Work out the finished part from the listing and answer in its coordinate system (mm). A direction names the side the tool comes from. Coordinates: 2 decimals unless noted, no trailing zeros. Write each loop counter-clockwise with the first axis right and the second up, starting at its lowest first coordinate (ties: lowest second). Pieces come first, ordered by that corner, then holes. Notation, with made-up numbers: (57, 24.25) - (62, 24.25) arc R35 ccw to (62, 57.25) - close; hole circle Ø10 at (-21.75, 39). An arc over 180 degrees is marked (long way). One line per item, written item: value.
```python
from build123d import *

# Parameters (mm, degrees)
ESQUISSE1_W              = 57
ESQUISSE1_H              = 57
BOSS_EXTRU_1_DEPTH       = 18.5
ESQUISSE2_W              = 51
ESQUISSE2_H              = 51
ENL_V_MAT_EXTRU_1_DEPTH  = 15.5
ESQUISSE4_W              = 10
ESQUISSE4_H              = 8
BOSS_EXTRU_2_DEPTH       = 10
ESQUISSE5_W              = 10
ESQUISSE5_H              = 8
BOSS_EXTRU_3_DEPTH       = 10
ESQUISSE6_W              = 10
ESQUISSE6_H              = 7
BOSS_EXTRU_4_DEPTH       = 10
ESQUISSE7_W              = 10
ESQUISSE7_H              = 7
BOSS_EXTRU_5_DEPTH       = 10
ESQUISSE8_R              = 1.7
ENL_V_MAT_EXTRU_2_DEPTH  = 12
ESQUISSE9_R              = 1.7
ENL_V_MAT_EXTRU_3_DEPTH  = 12
ESQUISSE16_R             = 1.7
ENL_V_MAT_EXTRU_9_DEPTH  = 12
ESQUISSE17_R             = 1.7
ENL_V_MAT_EXTRU_10_DEPTH = 12
ESQUISSE21_W             = 7.8
ESQUISSE21_H             = 2.8
ENL_V_MAT_EXTRU_14_DEPTH = 3
ENL_V_START              = -7.5
ENL_V_MAT_EXTRU_18_DEPTH = 2.7
ENL_V_MAT_EXTRU_20_DEPTH = 2.7
ESQUISSE26_W             = 5.54
ESQUISSE26_H             = 2.5
ENL_V_MAT_EXTRU_21_DEPTH = 2.847955181
ENL_V_MAT_EXTRU_22_DEPTH = 2.7
ENL_V_MAT_EXTRU_24_DEPTH = 2.7
ESQUISSE23_W             = 5.54
ESQUISSE23_H             = 2.5
ENL_V_MAT_EXTRU_26_DEPTH = 2
ESQUISSE31_W             = 5.54
ESQUISSE31_H             = 2.5
ENL_V_MAT_EXTRU_27_DEPTH = 2
ESQUISSE30_W             = 5.54
ESQUISSE30_H             = 2.5
ENL_V_MAT_EXTRU_28_DEPTH = 2
ESQUISSE32_W             = 57
ESQUISSE32_H             = 1
ENL_V_MAT_EXTRU_29_DEPTH = 0.5
ESQUISSE33_W             = 57
ESQUISSE33_H             = 1
ENL_V_MAT_EXTRU_30_DEPTH = 0.5
ESQUISSE34_W             = 57
ESQUISSE34_H             = 1
ENL_V_MAT_EXTRU_31_DEPTH = 0.5
ESQUISSE35_W             = 57
ESQUISSE35_H             = 1
ENL_V_MAT_EXTRU_32_DEPTH = 0.5
ESQUISSE36_W             = 11.4
ESQUISSE36_H             = 10.780005484
ENL_V_MAT_EXTRU_33_DEPTH = 2
CONG_1_R                 = 0.5
CONG_2_R                 = 0.5
CONG_3_R                 = 0.5
CONG_4_R                 = 0.5
CONG_5_R                 = 0.5
CONG_6_R                 = 0.5
CONG_7_R                 = 0.5
CONG_8_R                 = 0.5
CONG_9_R                 = 0.5
CONG_10_R                = 0.5
CONG_11_R                = 0.5
CONG_12_R                = 0.5
ESQUISSE38_W             = 28
ESQUISSE38_H             = 4.913001224
ENL_V_MAT_EXTRU_34_DEPTH = 3


with BuildPart() as part:
    # Esquisse1 → Boss.-Extru.1 (new body)
    with BuildSketch(Plane(origin=(0, 0, 0), x_dir=(1, 0, 0), z_dir=(0, 1, 0))):
        with Locations((-1.510072399, 8.394175698)):
            Rectangle(ESQUISSE1_W, ESQUISSE1_H)
    extrude(amount=BOSS_EXTRU_1_DEPTH)

    # Esquisse2 → Enlèv. mat.-Extru.1 (cut)
    with BuildSketch(Plane(origin=(0, 18.5, 0), x_dir=(1, 0, 0), z_dir=(0, 1, 0))):
        with Locations((-1.510072399, 8.394175698)):
            Rectangle(ESQUISSE2_W, ESQUISSE2_H)
    extrude(amount=-ENL_V_MAT_EXTRU_1_DEPTH, mode=Mode.SUBTRACT)

    # Esquisse4 → Boss.-Extru.2 (add)
    with BuildSketch(Plane(origin=(0, 3, 0), x_dir=(1, 0, 0), z_dir=(0, 1, 0))):
        with Locations((-22.010072399, 29.894175698)):
            Rectangle(ESQUISSE4_W, ESQUISSE4_H)
    extrude(amount=BOSS_EXTRU_2_DEPTH)

    # Esquisse5 → Boss.-Extru.3 (add)
    with BuildSketch(Plane(origin=(0, 3, 0), x_dir=(1, 0, 0), z_dir=(0, 1, 0))):
        with Locations((18.989927601, 29.894175698)):
            Rectangle(ESQUISSE5_W, ESQUISSE5_H)
    extrude(amount=BOSS_EXTRU_3_DEPTH)

    # Esquisse6 → Boss.-Extru.4 (add)
    with BuildSketch(Plane(origin=(0, 3, 0), x_dir=(1, 0, 0), z_dir=(0, 1, 0))):
        with Locations((18.989927601, -13.605824302)):
            Rectangle(ESQUISSE6_W, ESQUISSE6_H)
    extrude(amount=BOSS_EXTRU_4_DEPTH)

    # Esquisse7 → Boss.-Extru.5 (add)
    with BuildSketch(Plane(origin=(0, 3, 0), x_dir=(1, 0, 0), z_dir=(0, 1, 0))):
        with Locations((-22.010072399, -13.605824302)):
            Rectangle(ESQUISSE7_W, ESQUISSE7_H)
    extrude(amount=BOSS_EXTRU_5_DEPTH)

    # Esquisse8 → Enlèv. mat.-Extru.2 (cut)
    with BuildSketch(Plane(origin=(0, 13, 0), x_dir=(1, 0, 0), z_dir=(0, 1, 0))):
        with Locations(Location((19.489927601, -13.105824302, 0), (0, 0, 270))):
            Circle(ESQUISSE8_R)
    extrude(amount=-ENL_V_MAT_EXTRU_2_DEPTH, mode=Mode.SUBTRACT)

    # Esquisse9 → Enlèv. mat.-Extru.3 (cut)
    with BuildSketch(Plane(origin=(0, 13, 0), x_dir=(1, 0, 0), z_dir=(0, 1, 0))):
        with Locations(Location((-22.510072399, -13.105824302, 0), (0, 0, 270))):
            Circle(ESQUISSE9_R)
    extrude(amount=-ENL_V_MAT_EXTRU_3_DEPTH, mode=Mode.SUBTRACT)

    # Esquisse16 → Enlèv. mat.-Extru.9 (cut)
    with BuildSketch(Plane(origin=(0, 13, 0), x_dir=(1, 0, 0), z_dir=(0, 1, 0))):
        with Locations(Location((-22.510072399, 28.894175698, 0), (0, 0, 270))):
            Circle(ESQUISSE16_R)
    extrude(amount=-ENL_V_MAT_EXTRU_9_DEPTH, mode=Mode.SUBTRACT)

    # Esquisse17 → Enlèv. mat.-Extru.10 (cut)
    with BuildSketch(Plane(origin=(0, 13, 0), x_dir=(1, 0, 0), z_dir=(0, 1, 0))):
        with Locations(Location((19.489927601, 28.894175698, 0), (0, 0, 270))):
            Circle(ESQUISSE17_R)
    extrude(amount=-ENL_V_MAT_EXTRU_10_DEPTH, mode=Mode.SUBTRACT)

    # Esquisse21 → Enlèv. mat.-Extru.14 (cut)
    with BuildSketch(Plane.XY.offset(20.105824302)):
        with Locations((-1.510072399, 16.07)):
            Rectangle(ESQUISSE21_W, ESQUISSE21_H)
    extrude(amount=-ENL_V_MAT_EXTRU_14_DEPTH, mode=Mode.SUBTRACT)

    # Esquisse24 → Enlèv. mat.-Extru.18 (cut)
    with BuildSketch(Plane(origin=(0, 13, 0), x_dir=(1, 0, 0), z_dir=(0, 1, 0)).offset(ENL_V_START)):
        Polygon((19.489927601, 25.694175698), (22.261208893, 27.294175698), (22.261208893, 30.494175698), (19.489927601, 32.094175698), (16.718646309, 30.494175698), (16.718646309, 27.294175698), align=None)
    extrude(amount=-ENL_V_MAT_EXTRU_18_DEPTH, mode=Mode.SUBTRACT)

    # Esquisse25 → Enlèv. mat.-Extru.20 (cut)
    with BuildSketch(Plane(origin=(0, 13, 0), x_dir=(1, 0, 0), z_dir=(0, 1, 0)).offset(ENL_V_START)):
        Polygon((16.718646309, -11.505824302), (16.718646309, -14.705824302), (19.489927601, -16.305824302), (22.261208893, -14.705824302), (22.261208893, -11.505824302), (19.489927601, -9.905824302), align=None)
    extrude(amount=-ENL_V_MAT_EXTRU_20_DEPTH, mode=Mode.SUBTRACT)

    # Esquisse26 → Enlèv. mat.-Extru.21 (cut)
    with BuildSketch(Plane(origin=(0, 0, 10.105824302), x_dir=(-1, 0, 0), z_dir=(0, 0, -1))):
        with Locations((-19.489927601, 4.25)):
            Rectangle(ESQUISSE26_W, ESQUISSE26_H)
    extrude(amount=-ENL_V_MAT_EXTRU_21_DEPTH, mode=Mode.SUBTRACT)

    # Esquisse27 → Enlèv. mat.-Extru.22 (cut)
    with BuildSketch(Plane(origin=(0, 13, 0), x_dir=(1, 0, 0), z_dir=(0, 1, 0)).offset(ENL_V_START)):
        Polygon((-19.738791107, 27.294175698), (-19.738791107, 30.494175698), (-22.510072399, 32.094175698), (-25.281353691, 30.494175698), (-25.281353691, 27.294175698), (-22.510072399, 25.694175698), align=None)
    extrude(amount=-ENL_V_MAT_EXTRU_22_DEPTH, mode=Mode.SUBTRACT)

    # Esquisse29 → Enlèv. mat.-Extru.24 (cut)
    with BuildSketch(Plane(origin=(0, 13, 0), x_dir=(1, 0, 0), z_dir=(0, 1, 0)).offset(ENL_V_START)):
        Polygon((-19.738791107, -11.505824302), (-22.510072399, -9.905824302), (-25.281353691, -11.505824302), (-25.281353691, -14.705824302), (-22.510072399, -16.305824302), (-19.738791107, -14.705824302), align=None)
    extrude(amount=-ENL_V_MAT_EXTRU_24_DEPTH, mode=Mode.SUBTRACT)

    # Esquisse23 → Enlèv. mat.-Extru.26 (cut)
    with BuildSketch(Plane.XY.offset(-25.894175698)):
        with Locations((19.489927601, 4.25)):
            Rectangle(ESQUISSE23_W, ESQUISSE23_H)
    extrude(amount=-ENL_V_MAT_EXTRU_26_DEPTH, mode=Mode.SUBTRACT)

    # Esquisse31 → Enlèv. mat.-Extru.27 (cut)
    with BuildSketch(Plane.XY.offset(-25.894175698)):
        with Locations((-22.510072399, 4.25)):
            Rectangle(ESQUISSE31_W, ESQUISSE31_H)
    extrude(amount=-ENL_V_MAT_EXTRU_27_DEPTH, mode=Mode.SUBTRACT)

    # Esquisse30 → Enlèv. mat.-Extru.28 (cut)
    with BuildSketch(Plane(origin=(0, 0, 10.105824302), x_dir=(-1, 0, 0), z_dir=(0, 0, -1))):
        with Locations((22.510072399, 4.25)):
            Rectangle(ESQUISSE30_W, ESQUISSE30_H)
    extrude(amount=-ENL_V_MAT_EXTRU_28_DEPTH, mode=Mode.SUBTRACT)

    # Esquisse32 → Enlèv. mat.-Extru.29 (cut)
    with BuildSketch(Plane.ZY.offset(30.010072399)):
        with Locations((-8.394175698, 8.219994516)):
            Rectangle(ESQUISSE32_W, ESQUISSE32_H)
    extrude(amount=-ENL_V_MAT_EXTRU_29_DEPTH, mode=Mode.SUBTRACT)

    # Esquisse33 → Enlèv. mat.-Extru.30 (cut)
    with BuildSketch(Plane.XY.offset(20.105824302)):
        with Locations((-1.510072399, 8.219994516)):
            Rectangle(ESQUISSE33_W, ESQUISSE33_H)
    extrude(amount=-ENL_V_MAT_EXTRU_30_DEPTH, mode=Mode.SUBTRACT)

    # Esquisse34 → Enlèv. mat.-Extru.31 (cut)
    with BuildSketch(Plane(origin=(26.989927601, 0, 0), x_dir=(0, 0, -1), z_dir=(1, 0, 0))):
        with Locations((8.394175698, 8.219994516)):
            Rectangle(ESQUISSE34_W, ESQUISSE34_H)
    extrude(amount=-ENL_V_MAT_EXTRU_31_DEPTH, mode=Mode.SUBTRACT)

    # Esquisse35 → Enlèv. mat.-Extru.32 (cut)
    with BuildSketch(Plane(origin=(0, 0, -36.894175698), x_dir=(-1, 0, 0), z_dir=(0, 0, -1))):
        with Locations((1.510072399, 8.219994516)):
            Rectangle(ESQUISSE35_W, ESQUISSE35_H)
    extrude(amount=-ENL_V_MAT_EXTRU_32_DEPTH, mode=Mode.SUBTRACT)

    # Esquisse36 → Enlèv. mat.-Extru.33 (cut)
    with BuildSketch(Plane.XY.offset(20.105824302)):
        with Locations((-1.510072399, 13.109997258)):
            Rectangle(ESQUISSE36_W, ESQUISSE36_H)
    extrude(amount=-ENL_V_MAT_EXTRU_33_DEPTH, mode=Mode.SUBTRACT)

    # Congé1
    cong_1_edges = [part.edges().sort_by_distance(p)[0] for p in [
        (-7.210072399, 13.609997258, 20.105824302),
    ]]
    fillet(cong_1_edges, radius=CONG_1_R)

    # Congé2
    cong_2_edges = [part.edges().sort_by_distance(p)[0] for p in [
        (4.189927601, 13.609997258, 20.105824302),
    ]]
    fillet(cong_2_edges, radius=CONG_2_R)

    # Congé3
    cong_3_edges = [part.edges().sort_by_distance(p)[0] for p in [
        (-7.210072399, 8.219994516, 19.605824302),
    ]]
    fillet(cong_3_edges, radius=CONG_3_R)

    # Congé4
    cong_4_edges = [part.edges().sort_by_distance(p)[0] for p in [
        (4.189927601, 8.219994516, 19.605824302),
    ]]
    fillet(cong_4_edges, radius=CONG_4_R)

    # Congé5
    cong_5_edges = [part.edges().sort_by_distance(p)[0] for p in [
        (26.989927601, 13.609997258, 20.105824302),
    ]]
    fillet(cong_5_edges, radius=CONG_5_R)

    # Congé6
    cong_6_edges = [part.edges().sort_by_distance(p)[0] for p in [
        (26.989927601, 3.859997258, 20.105824302),
    ]]
    fillet(cong_6_edges, radius=CONG_6_R)

    # Congé7
    cong_7_edges = [part.edges().sort_by_distance(p)[0] for p in [
        (26.989927601, 13.609997258, -36.894175698),
    ]]
    fillet(cong_7_edges, radius=CONG_7_R)

    # Congé8
    cong_8_edges = [part.edges().sort_by_distance(p)[0] for p in [
        (26.989927601, 3.859997258, -36.894175698),
    ]]
    fillet(cong_8_edges, radius=CONG_8_R)

    # Congé9
    cong_9_edges = [part.edges().sort_by_distance(p)[0] for p in [
        (-30.010072399, 13.609997258, -36.894175698),
    ]]
    fillet(cong_9_edges, radius=CONG_9_R)

    # Congé10
    cong_10_edges = [part.edges().sort_by_distance(p)[0] for p in [
        (-30.010072399, 3.859997258, -36.894175698),
    ]]
    fillet(cong_10_edges, radius=CONG_10_R)

    # Congé11
    cong_11_edges = [part.edges().sort_by_distance(p)[0] for p in [
        (-30.010072399, 13.609997258, 20.105824302),
    ]]
    fillet(cong_11_edges, radius=CONG_11_R)

    # Congé12
    cong_12_edges = [part.edges().sort_by_distance(p)[0] for p in [
        (-30.010072399, 3.859997258, 20.105824302),
    ]]
    fillet(cong_12_edges, radius=CONG_12_R)

    # Esquisse38 → Enlèv. mat.-Extru.34 (cut)
    with BuildSketch(Plane(origin=(0, 0, -36.894175698), x_dir=(-1, 0, 0), z_dir=(0, 0, -1))):
        with Locations((1.510072399, 7.254987661)):
            Rectangle(ESQUISSE38_W, ESQUISSE38_H)
    extrude(amount=-ENL_V_MAT_EXTRU_34_DEPTH, mode=Mode.SUBTRACT)


solid = part.part
```
Item 1: Consider probe 1 along Z at (x, y) = (16.5, 11.75); probe 2 along X at (y, z) = (15, -30); probe 3 along X at (y, z) = (7.75, -11.5). Determine where each line is inside the solid, lowest interval first.
Evaluation:
probe 1: z = -36.89 to -25.89, 10.11 to 20.11
probe 2: x = -30.01 to -27.01, 23.99 to 26.99
probe 3: x = -29.51 to -27.01, 23.99 to 26.49
Item 2: Section A-A, the plane x = -10 is taken. Determine the outline of the cut face in (y, z).
Evaluation:
outline: (0, -36.89) - (4.8, -36.89) - (4.8, -33.89) - (3, -33.89) - (3, 17.11) - (18.5, 17.11) - (18.5, 20.11) - (8.72, 20.11) - (8.72, 19.61) - (7.72, 19.61) - (7.72, 20.11) - (0, 20.11) - close; (9.71, -36.89) - (18.5, -36.89) - (18.5, -33.89) - (9.71, -33.89) - close
Item 3: Determine the mould class of faces 5 (the face through (17.8, 13, 14.3)), 6 (the face through (18.456, 9.302, 11.757)), 7 (the face through (16.719, 4, -29)) for opening direction Y: +Y half, -Y half, draft (parallel to the pull), parting line (faces both ways), or undercut.
Evaluation:
face 5: +Y half
face 6: draft
face 7: undercut
Item 4: Given pin 1 (5 mm diameter, centred on y = 8.5, z = 4, fed in from -X); pin 2 (1 mm diameter, centred on x = 6, z = 3.5, fed in from +Y); pin 3 (0.5 mm diameter, centred on y = 8, z = -17.5, fed in from -X), each flat-ended and moving along its own axis, determine where each tip first touches the part or whether it passes through.
Evaluation:
pin 1: stops at x = -30.01
pin 2: stops at y = 3
pin 3: stops at x = -29.51
Item 5: Which of the six approach directions +Z, -Z, +X, -X, +Y, -Y give full straight-line access (tool end or side, diameter ignored) to faces 1 (the face through (-2, 14, -36.894)), 2 (the face through (-1, 4.798, -35)), 3 (the face through (20, 1, 13)), 4 (the face through (20.895, 4.169, -31.283))?
Evaluation:
face 1: -Z, +X, -X, +Y, -Y
face 2: -Z
face 3: +Y
face 4: none
Item 6: Section B-B, the plane y = 11.25 is taken. Give the number of separate pieces and of enclosed holes in the cut face, then the cut area to 3 significant figures.
Evaluation:
separate pieces: 1
enclosed holes: 5
area: 889 mm2
Item 7: Section C-C, the plane z = 9 is taken. Determine the outline of the cut face in (x, y).
Evaluation:
outline: (-30.01, 0) - (26.99, 0) - (26.99, 7.72) - (26.49, 7.72) - (26.49, 8.72) - (26.99, 8.72) - (26.99, 18.5) - (23.99, 18.5) - (23.99, 3) - (-27.01, 3) - (-27.01, 18.5) - (-30.01, 18.5) - (-30.01, 8.72) - (-29.51, 8.72) - (-29.51, 7.72) - (-30.01, 7.72) - close
Item 8: Section D-D, the plane x = 16 is taken. Determine the outline of the cut face in (y, z), then the cut area to 3 significant figures.
Evaluation:
outline: (0, -36.89) - (7.72, -36.89) - (7.72, -36.39) - (8.72, -36.39) - (8.72, -36.89) - (18.5, -36.89) - (18.5, -33.89) - (13, -33.89) - (13, -25.89) - (3, -25.89) - (3, 10.11) - (13, 10.11) - (13, 17.11) - (18.5, 17.11) - (18.5, 20.11) - (8.72, 20.11) - (8.72, 19.61) - (7.72, 19.61) - (7.72, 20.11) - (0, 20.11) - close
area: 413 mm2
